Drawing for the job (mm, zero at the part's lowest x, y, z). A direction names the side the tool comes from. Round coordinates to 2 decimals unless told otherwise and drop trailing zeros. Write each loop counter-clockwise with the first axis right and the second up, starting at its lowest first coordinate (ties: lowest second). Pieces come first, ordered by that corner, then holes.
Item 1: Drop flat-ended pins along their axis: pin 1 Ø1.5 at (x, y) = (80, 3) entering from +Z; pin 2 Ø4.5 at (y, z) = (1.5, 19.5) entering from -X; pin 3 Ø10 at (y, z) = (6.5, 97.5) entering from +X. Give the stop position or say it passes through.
Item 2: Band-saw the part on C-C, the plane x = 39.5. Write the cut outline in (y, z), then the cut area to 3 significant figures.
Item 3: Band-saw the part on D-D, the plane z = 51.5. Write the cut outline in (x, y), then the cut area to 3 significant figures.
Item 4: Band-saw the part on B-B, the plane y = 12. Write the cut outline in (x, z), then the cut area to 3 significant figures.
Item 5: Band-saw the part on A-A, the plane z = 16. Write the cut outline in (x, y).
Item 6: Wall check: probe 1 along X at (y, z) = (1.75, 12.5); probe 2 along Y at (x, z) = (92, 5); probe 3 along X at (y, z) = (12.5, 19). Give the ranges that are in metal, low to high.
Item 7: 3-axis set-ups, long thin cutter, end or side, ignore diameter. For the marked faces 1, 2 and 3: which of +Z, -Z, +X, -X, +Y, -Y reach the whole face in a straight line?
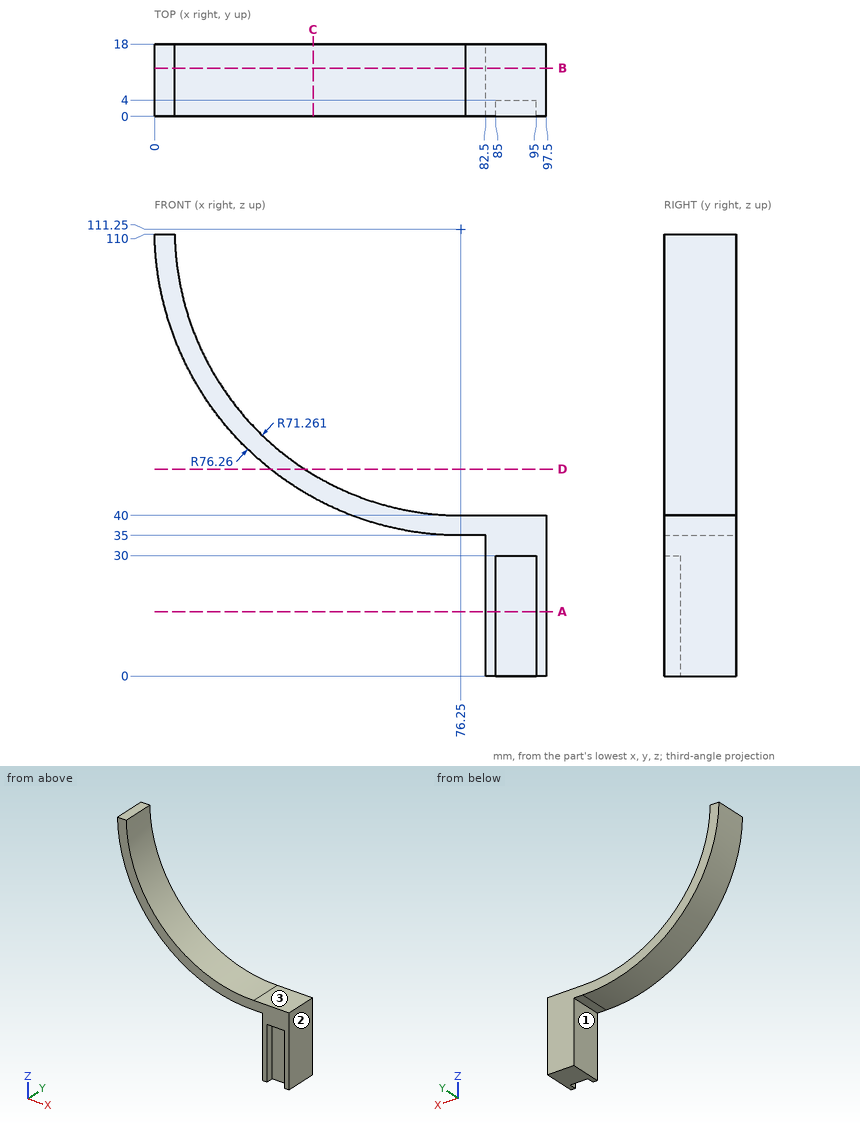
Results:
1. pin 1: stops at z = 40
1. pin 2: stops at x = 82.5
1. pin 3: stops at x = 7.5
2. outline: (0, 44.43) - (18, 44.43) - (18, 50.2) - (0, 50.2) - close
2. area: 104 mm2
3. outline: (28.86, 0) - (37.42, 0) - (37.42, 18) - (28.86, 18) - close
3. area: 154 mm2
4. outline: (0, 110) arc R76.26 ccw to (77.5, 35) - (82.5, 35) - (82.5, 0) - (97.5, 0) - (97.5, 40) - (77.5, 40) arc R71.26 cw to (5, 110) - close
4. area: 1,200 mm2
5. outline: (82.5, 0) - (85, 0) - (85, 4) - (95, 4) - (95, 0) - (97.5, 0) - (97.5, 18) - (82.5, 18) - close
6. probe 1: x = 82.5 to 85, 95 to 97.5
6. probe 2: y = 4 to 18
6. probe 3: x = 82.5 to 97.5
7. face 1: -Z, -X, +Y, -Y
7. face 2: +Z, -Z, +X, +Y, -Y
7. face 3: +Z, +X, +Y, -Y
